```python
from build123d import *

# Parameters (mm, degrees)
SKETCH11_W         = 114.3
SKETCH11_H         = 44.45
SKETCH11_R         = 6.36905
SKETCH11_R_2       = 7.94385
EXTRUDE3_DEPTH     = 15.875
CUT_EXTRUDE1_DEPTH = 30.226
FILLET1_R          = 12.7
EXTRUDE4_DEPTH     = 5.9944
SKETCH15_R         = 24.22520922
CUT_EXTRUDE2_DEPTH = 12.9888


with BuildPart() as part:
    # Sketch11 → Extrude3 (new body, symmetric)
    with BuildSketch(Plane.XY):
        with Locations((-44.45, 9.525)):
            Rectangle(SKETCH11_W, SKETCH11_H)
        Circle(SKETCH11_R, mode=Mode.SUBTRACT)
        with Locations((-44.45, 6.35)):
            Circle(SKETCH11_R_2, mode=Mode.SUBTRACT)
    extrude(amount=EXTRUDE3_DEPTH, both=True)

    # Sketch12 → Cut-Extrude1 (cut)
    with BuildSketch(Plane.XZ.offset(12.7)):
        with BuildLine():
            Line((-17.526, 8.0645), (12.7, 8.0645))
            Line((12.7, 8.0645), (12.7, -8.0645))
            Line((12.7, -8.0645), (-17.526, -8.0645))
            ThreePointArc((-17.526, -8.0645), (-25.5905, 0), (-17.526, 8.0645))
        make_face()
    extrude(amount=-CUT_EXTRUDE1_DEPTH, mode=Mode.SUBTRACT)

    # Fillet1
    fillet1_edges = [part.edges().sort_by_distance(p)[0] for p in [
        (12.7, -12.7, -11.96975),
        (12.7, 31.75, 0),
        (12.7, -12.7, 11.96975),
    ]]
    fillet(fillet1_edges, radius=FILLET1_R)

    # Sketch13 → Extrude4 (add)
    with BuildSketch(Plane(origin=(0, 31.75, 0), x_dir=(1, 0, 0), z_dir=(0, 1, 0))):
        Polygon((-78.502729942, 0), (-83.701364971, 9.0043), (-94.098635029, 9.0043), (-99.297270058, 0), (-94.098635029, -9.0043), (-83.701364971, -9.0043), align=None)
    extrude(amount=EXTRUDE4_DEPTH)

    # Sketch14 → Revolve2 (revolve)
    with BuildSketch(Plane.XY, mode=Mode.PRIVATE) as revolve2_sk:
        with BuildLine():
            Line((-93.8022, 66.5988), (-93.8022, 69.85))
            Line((-93.8022, 69.85), (-88.9, 69.85))
            Line((-88.9, 69.85), (-88.9, -25.4))
            ThreePointArc((-88.9, -25.4), (-102.250110486, -22.456892404), (-113.12520922, -14.1732))
            Line((-113.12520922, -14.1732), (-113.12520922, -13.4112))
            Line((-113.12520922, -13.4112), (-94.8944, -13.4112))
            Line((-94.8944, -13.4112), (-94.8944, 65.5066))
            Line((-94.8944, 65.5066), (-93.8022, 66.5988))
        make_face()
    revolve(revolve2_sk.sketch.rotate(Axis((-88.9, 71.228986791, 0), (0, -1, 0)), 270), axis=Axis((-88.9, 71.228986791, 0), (0, -1, 0)))  # turned: the seam where the file's is

    # Sketch15 → Cut-Extrude2 (cut, through all)
    with BuildSketch(Plane(origin=(0, -13.4112, 0), x_dir=(1, 0, 0), z_dir=(0, 1, 0))):
        with Locations((-88.9, 0)):
            Circle(SKETCH15_R)
        Polygon((-88.9, 8.477361778), (-97.377361778, 0), (-88.9, -8.477361778), (-80.422638222, 0), align=None, mode=Mode.SUBTRACT)
    extrude(amount=-CUT_EXTRUDE2_DEPTH, mode=Mode.SUBTRACT)


solid = part.part
```
Check sheet for the modelled part. Datum: model origin and axes. Units: mm. A direction names the side the tool comes from. Round coordinates to 2 decimals unless told otherwise and drop trailing zeros. Order: outer loops, then holes, each group sorted by start corner. A loop starts at its lowest first (then second) coordinate and runs counter-clockwise, first axis right, second up. Notation, with made-up numbers: (-25.75, 76) -> (23.25, 76) arc R23 cw to (23.25, 85) -> close; hole circle Ø5 at (-9, -7.5). An arc over 180 degrees is marked (long way). One line per item, written item: value. Start each with the question number.
Q1. Cross-section at D-D (x = -29). Record the boundary of the cut face in (y, z) (3 decimals).
Q2. Gauge pin test, flat ends, axial feed: pin 1 Ø5 at (x, y) = (-91, 35.5) entering from +Z; pin 2 Ø17.5 at (x, z) = (-14.5, 2) entering from -Y; pin 3 Ø2 at (x, z) = (-90, -6.5) entering from +Y. Record the tip position at first contact, or that the pin passes through.
Q3. Cross-section at B-B (z = -11). Record the boundary of the cut face in (x, y), and give its area (3 significant figures).
Q4. Cross-section at A-A (x = -44.45). Record the boundary of the cut face in (y, z) (3 decimals).
Q5. Set-up check for faces 4 (the face through (-81.066, 34.705, -4.439)), 5 (the face through (-6, 17.526, 0)), 6 (the face through (-84.6, -19.04, -4.18)), 7 (the face through (-89, 35, -9.004)): record each of +Z, -Z, +X, -X, +Y, -Y from which the full face is reachable in a straight line by a thin tool's end or side.
Q6. Cross-section at C-C (y = 8.5). Record the boundary of the cut face in (x, z) (1 decimal).
Q7. Mould release check, pull along X, two halves, no side actions. Record for faces 1 (the face through (-83.05, 51.82, -1.3)), 2 (the face through (-5.05, -3.88, -12.02)), 3 (the face through (-45, 15, 15.875)): pulls with the +X half, pulls with the -X half, needs draft (parallel to the pull), parting line crosses it, or undercut.
Q8. Thickness scan on line 1 (Y direction, x = 0, z = -10); line 2 (Y direction, x = -44.45, z = 9.5); line 3 (X direction, y = 0, z = -11). Record the ranges inside material, lowest first.
Completed:
1. outline: (-12.7, -15.875) -> (31.75, -15.875) -> (31.75, 15.875) -> (-12.7, 15.875) -> close
2. pin 1: stops at z = 9
2. pin 2: stops at y = -12.7
2. pin 3: stops at y = 65.91
3. outline: (-101.6, -12.7) -> (0, -12.7) arc R12.7 ccw to (12.7, 0) -> (12.7, 19.05) arc R12.7 ccw to (0, 31.75) -> (-101.6, 31.75) -> close; hole circle Ø15.89 at (-44.45, 6.35); hole circle Ø12.74 at (0, 0)
3. area: 4,690 mm²
4. outline: (-12.7, -15.875) -> (-1.594, -15.875) -> (-1.594, 15.875) -> (-12.7, 15.875) -> close; (14.294, -15.875) -> (31.75, -15.875) -> (31.75, 15.875) -> (14.294, 15.875) -> close
5. face 4: -Z, +X, +Y
5. face 5: +X, -Y
5. face 6: -Z, +X, -Y
5. face 7: -Z, +X, -X, +Y
6. outline: (-101.6, -15.9) -> (-52.1, -15.9) -> (-52.1, 15.9) -> (-101.6, 15.9) -> close; (-36.8, -15.9) -> (12.7, -15.9) -> (12.7, -8.1) -> (-17.5, -8.1) arc R8.1 cw to (-17.5, 8.1) -> (12.7, 8.1) -> (12.7, 15.9) -> (-36.8, 15.9) -> close
7. face 1: parting line crosses it
7. face 2: undercut
7. face 3: needs draft
8. line 1: y = -12.7 to -6.37, 6.37 to 31.75
8. line 2: y = -12.7 to -1.59, 14.29 to 31.75
8. line 3: x = -101.6 to -49.22, -39.68 to -6.37, 6.37 to 12.7
